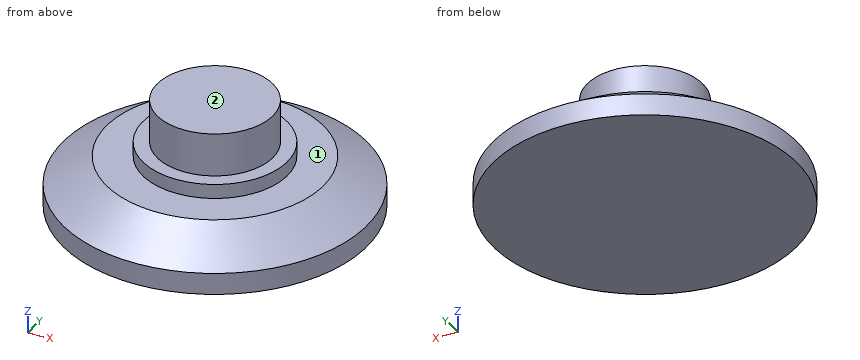
from build123d import *

# Parameters (mm, degrees)
F0_R     = 10.5
F1_DEPTH = 3.5
F2_R     = 5
F3_DEPTH = 1
F4_R     = 4
F5_DEPTH = 3
F6_SIZE2 = 2
F6_SIZE  = 3


with BuildPart() as f1:
    # F0 (on Top) → F1 (new body)
    with BuildSketch(Plane.XY):
        Circle(F0_R)
    extrude(amount=F1_DEPTH)

    # F2 (on face) → F3 (join)
    with BuildSketch(Plane.XY.offset(3.5)):
        Circle(F2_R)
    extrude(amount=F3_DEPTH)

    # F4 (on face) → F5 (join)
    with BuildSketch(Plane.XY.offset(4.5)):
        Circle(F4_R)
    extrude(amount=F5_DEPTH)

    # F6
    f6_edges = [f1.edges().sort_by_distance(p)[0] for p in [
        (-10.5, 0, 3.5),
    ]]
    f6_side = f1.faces().sort_by_distance((-10.203015, 0, 3.5))[0]
    chamfer(f6_edges, length=F6_SIZE, length2=F6_SIZE2, reference=f6_side)


solid = f1.part
Verification items for the finished model (mm, model axes). Face numbers are marked on the shaded views. A direction names the side the tool comes from. Give positions to 0.01 mm unless a question says otherwise; leave off trailing zeros. Order: outer loops, then holes, each group sorted by start corner. A loop starts at its lowest first (then second) coordinate and runs counter-clockwise, first axis right, second up. Notation, with made-up numbers: M 19,57.5 L 66,57.5 A28 ccw 66,77.5 Z; hole C -18.5,68 d11. An arc over 180 degrees is marked long. Answer as a JSON object with one key per item and string values. Group by question number.
1) Access from +Z, -Z, +X, -X, +Y, -Y to the whole of each face (thin tool, end or side, straight path). Record for the marked faces 1 and 2.
2) Depth check by flat-ended pin: pin 1 Ø1 at (x, y) = (4, 4.5) entering from +Z; pin 2 Ø1 at (x, z) = (4.5, 3) entering from +Y; pin 3 Ø3 at (y, z) = (5.5, 1) entering from +X. Enter the tip coordinate at first touch or a pass-through.
3) Cross-section at D-D (z = 7.25). Enter the section's corners in (x, y), then the cut area to 3 significant figures.
4) Cross-section at A-A (x = 0). Enter the section's corners in (y, z).
5) Scan lines: line 1 along Z through (x, y) = (-7, 2); line 2 along Z through (x, y) = (4, 1.25); line 3 along Y through (x, z) = (-2.75, 0.75). Record each from-to range of solid material in increasing order. Write a range as [from, to].
6) Cross-section at C-C (z = 4). Enter the section's corners in (x, y).
Result sheet:
{
 "1": {"face 1": "+Z", "face 2": "+Z, +X, -X, +Y, -Y"},
 "2": {"pin 1": "stops at z = 3.5", "pin 2": "stops at y = 7.84", "pin 3": "stops at x = 9.71"},
 "3": {"outline": "C 0,0 d8", "area": "50.3 mm2"},
 "4": {"outline": "M -10.5,0 L 10.5,0 L 10.5,1.5 L 7.5,3.5 L 5,3.5 L 5,4.5 L 4,4.5 L 4,7.5 L -4,7.5 L -4,4.5 L -5,4.5 L -5,3.5 L -7.5,3.5 L -10.5,1.5 Z"},
 "5": {"line 1": "z = [0, 3.5]", "line 2": "z = [0, 4.5]", "line 3": "y = [-10.13, 10.13]"},
 "6": {"outline": "C 0,0 d10"}
}
